For this review, take the finished solid that the model builds, in its own axes (mm). A direction names the side the tool comes from. Coordinates: 2 decimals unless noted, no trailing zeros. Order: outer loops, then holes, each group sorted by start corner. A loop starts at its lowest first (then second) coordinate and runs counter-clockwise, first axis right, second up. Notation, with made-up numbers: (-27.75, 17) -> (26.25, 17) arc R9 ccw to (26.25, 34) -> close; hole circle Ø3 at (48, 77). An arc over 180 degrees is marked (long way). Answer as a JSON object with one key per item and string values. Group by question number.
1) Add section A-A, the plane y = 94.5. Write out the cut boundary in (x, z), then the cut area to 3 significant figures.
2) Machinability: for faces 1 (the cylindrical face through (5, 94.9, 11)), 2 (the cylindrical face through (94.9, 5, 11)), 3 (the cylindrical face through (5, 5.1, 11)), 4 (the cylindrical face through (95, 94.9, 11)), 5 (the flat face through (50, 2, 10)), which of the approach directions +Z, -Z, +X, -X, +Y, -Y give a long, thin tool a straight path to every point of the face, cutting with its end or side? Answer none if there is none.
3) Wall thickness on L1, parallel to X at y = 18.5, z = 11.5; L2, parallel to X at y = 6.5, z = 8: over which ranges is each line inside the solid? List them lowest first.
4) For pin 1 (1.6 mm diameter, centred on x = 52, z = 11.5, fed in from -Y), flat-tipped, find the tip position at first contact; note if it passes through.
from build123d import *

# Parameters (mm, degrees)
BOX002_W     = 100
BOX002_H     = 100
BOX002_DEPTH = 10
FILLET002_R  = 7
BOX003_W     = 94
BOX003_H     = 94
BOX003_DEPTH = 2
FILLET003_R  = 7


with BuildPart() as body_with_fillets001:
    # Box002 → Box002 (new body)
    with BuildSketch(Plane.XY):
        with Locations((50, 50)):
            Rectangle(BOX002_W, BOX002_H)
    extrude(amount=BOX002_DEPTH)

    # Fillet002
    fillet002_edges = [body_with_fillets001.edges().sort_by_distance(p)[0] for p in [
        (0, 0, 5),
        (0, 100, 5),
        (100, 0, 5),
        (100, 100, 5),
    ]]
    fillet(fillet002_edges, radius=FILLET002_R)


with BuildPart() as base003:
    # Box003 → Box003 (new body)
    with BuildSketch(Plane(origin=(3, 3, 10), x_dir=(1, 0, 0), z_dir=(0, 0, 1))):
        with Locations((47, 47)):
            Rectangle(BOX003_W, BOX003_H)
    extrude(amount=BOX003_DEPTH)

    # Fillet003
    fillet003_edges = [base003.edges().sort_by_distance(p)[0] for p in [
        (3, 3, 11),
        (3, 97, 11),
        (97, 3, 11),
        (97, 97, 11),
    ]]
    fillet(fillet003_edges, radius=FILLET003_R)

    # Fusion001: union Body with fillets001
    add(body_with_fillets001.part)


solid = base003.part
Output values:
{
 "1": {"outline": "(0.16, 0) -> (99.84, 0) -> (99.84, 10) -> (95.36, 10) -> (95.36, 12) -> (4.64, 12) -> (4.64, 10) -> (0.16, 10) -> close", "area": "1,180 mm²"},
 "2": {"face 1": "+Z, -X, +Y", "face 2": "+Z, +X, -Y", "face 3": "+Z, -X, -Y", "face 4": "+Z, +X, +Y", "face 5": "+Z"},
 "3": {"L1": "x = 3 to 97", "L2": "x = 0.02 to 99.98"},
 "4": {"pin 1": "stops at y = 3"}
}
